Geometry check sheet. Reference: the model listing, model coordinates, mm. Round coordinates to 2 decimals unless told otherwise and drop trailing zeros. Write each loop counter-clockwise with the first axis right and the second up, starting at its lowest first coordinate (ties: lowest second). Pieces come first, ordered by that corner, then holes. Notation, with made-up numbers: M 34.5,-31.5 L 64.5,-31.5 A5 ccw 64.5,-24.5 Z; hole C 62,-11 d10. An arc over 180 degrees is marked long. One line per item, written item: value. Start each with the question number.
1. Scan lines: probe 1 along Z at (x, y) = (8.89, -2) (3 decimals); probe 2 along Z at (x, y) = (0, -1.95) (3 decimals); probe 3 along X at (y, z) = (-0.25, 34.5). Record each from-to range of solid material in increasing order. Write a range as [from, to].
2. Section check B-B (z = -34.5). Record the boundary of the cut face in (x, y) (3 decimals), and give its area (3 significant figures).
3. Section check C-C (x = -15). Record the boundary of the cut face in (y, z) (3 decimals), and give its area (3 significant figures).
4. Depth check by flat-ended pin: P1, Ø1.9, axis at x = 8.89, z = -36.83, coming from the -Y side (3 decimals); P2, Ø1, axis at y = -1.5, z = -30.5, coming from the +X side; P3, Ø1.6, axis at y = -1.5, z = 41, coming from the -X side; P4, Ø1.6, axis at x = 7, y = -1.5, coming from the +Z side (3 decimals). Enter the tip coordinate at first touch or a pass-through.
5. Section check A-A (y = -0.75). Record the boundary of the cut face in (x, z) (3 decimals), and give its area (3 significant figures).
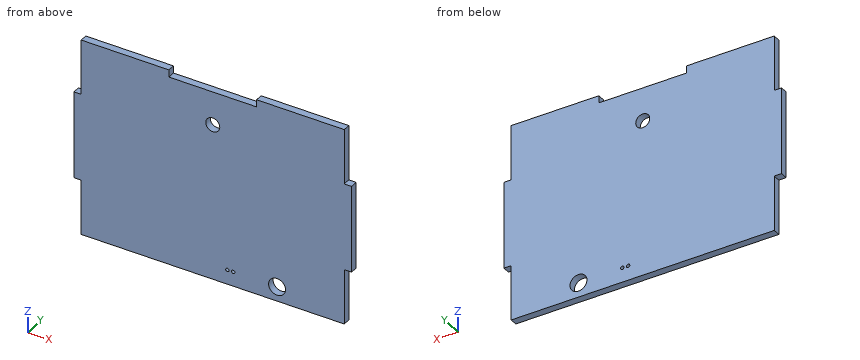
from build123d import *

# Parameters (mm, degrees)
F1_DEPTH = 3.175
F2_R     = 3.048
F2_R_2   = 3.683
F2_R_3   = 0.7366
F3_DEPTH = 3.176


# Not quite as in the source:
# - a feature names something its author has since deleted; it is built from what else it names


with BuildPart() as f1:
    # F0 (on Front) → F1 (new body)
    with BuildSketch(Plane.XZ):
        Polygon((-57.15, -43.18), (57.15, -43.18), (57.15, -19.05), (60.325, -19.05), (60.325, 19.05), (57.15, 19.05), (57.15, 43.18), (19.05, 43.18), (19.05, 40.005), (-19.05, 40.005), (-19.05, 43.18), (-57.15, 43.18), (-57.15, 19.05), (-60.325, 19.05), (-60.325, 0), (-60.325, -19.05), (-57.15, -19.05), align=None)
    extrude(amount=F1_DEPTH)

    # F2 (on face) → F3 (cut, through all)
    with BuildSketch(Plane.XZ.offset(3.175)):
        with Locations((0, 25.4)):
            Circle(F2_R)
        with Locations((27.94, -36.83)):
            Circle(F2_R_2)
        with Locations((6.35, -36.83)):
            Circle(F2_R_3)
        with Locations((8.89, -36.83)):
            Circle(F2_R_3)
    extrude(amount=-F3_DEPTH, mode=Mode.SUBTRACT)


solid = f1.part
Result sheet:
1. probe 1: z = [-43.18, -37.567], [-36.093, 40.005]
1. probe 2: z = [-43.18, 22.352], [28.448, 40.005]
1. probe 3: x = [-57.15, 57.15]
2. outline: M -57.15,-3.175 L 25.088,-3.175 L 25.088,0 L -57.15,0 Z; M 30.792,-3.175 L 57.15,-3.175 L 57.15,0 L 30.792,0 Z
2. area: 345 mm2
3. outline: M -3.175,-43.18 L 0,-43.18 L 0,40.005 L -3.175,40.005 Z
3. area: 264 mm2
4. P1: stops at y = -3.175
4. P2: stops at x = 57.15
4. P3: stops at x = -57.15
4. P4: stops at z = 40.005
5. outline: M -60.325,-19.05 L -57.15,-19.05 L -57.15,-43.18 L 57.15,-43.18 L 57.15,-19.05 L 60.325,-19.05 L 60.325,19.05 L 57.15,19.05 L 57.15,43.18 L 19.05,43.18 L 19.05,40.005 L -19.05,40.005 L -19.05,43.18 L -57.15,43.18 L -57.15,19.05 L -60.325,19.05 Z; hole C 0,25.4 d6.096; hole C 6.35,-36.83 d1.473; hole C 8.89,-36.83 d1.473; hole C 27.94,-36.83 d7.366
5. area: 9,920 mm2
